Can you work these out from the model? Positions are in its coordinate system, mm. Give positions to 0.01 mm unless a question says otherwise; leave off trailing zeros. Order: outer loops, then holes, each group sorted by start corner. A loop starts at its lowest first (then second) coordinate and runs counter-clockwise, first axis right, second up. Notation, with made-up numbers: M -16.5,40 L 33.5,40 A21 ccw 33.5,75 Z; hole C 59,-30 d7. An arc over 180 degrees is marked long. Write each question's results on one line, items separated by ' | '.
from build123d import *

# Parameters (mm, degrees)
SKETCH1_W           = 34
SKETCH1_H           = 26
BOSS_EXTRUDE1_DEPTH = 1.5
SKETCH2_R           = 1.5
CUT_EXTRUDE1_DEPTH  = 1.5
CHAMFER1_SIZE       = 1


with BuildPart() as part:
    # Sketch1 → Boss-Extrude1 (new body)
    with BuildSketch(Plane(origin=(0, 0, 0), x_dir=(1, 0, 0), z_dir=(0, 1, 0))):
        Rectangle(SKETCH1_W, SKETCH1_H)
    extrude(amount=BOSS_EXTRUDE1_DEPTH)

    # Sketch2 → Cut-Extrude1 (cut)
    with BuildSketch(Plane(origin=(0, 1.5, 0), x_dir=(1, 0, 0), z_dir=(0, 1, 0))):
        with Locations(Location((-14.5, 10.5, 0), (0, 0, 270))):
            Circle(SKETCH2_R)
        with Locations(Location((11.5, 10.5, 0), (0, 0, 270))):
            Circle(SKETCH2_R)
        with Locations(Location((11.5, -10.5, 0), (0, 0, 270))):
            Circle(SKETCH2_R)
        with Locations(Location((-14.5, -10.5, 0), (0, 0, 270))):
            Circle(SKETCH2_R)
    extrude(amount=-CUT_EXTRUDE1_DEPTH, mode=Mode.SUBTRACT)

    # Chamfer1
    chamfer1_edges = [part.edges().sort_by_distance(p)[0] for p in [
        (17, 0.75, 13),
        (-17, 0.75, 13),
        (-17, 0.75, -13),
        (17, 0.75, -13),
    ]]
    chamfer(chamfer1_edges, length=CHAMFER1_SIZE)


solid = part.part
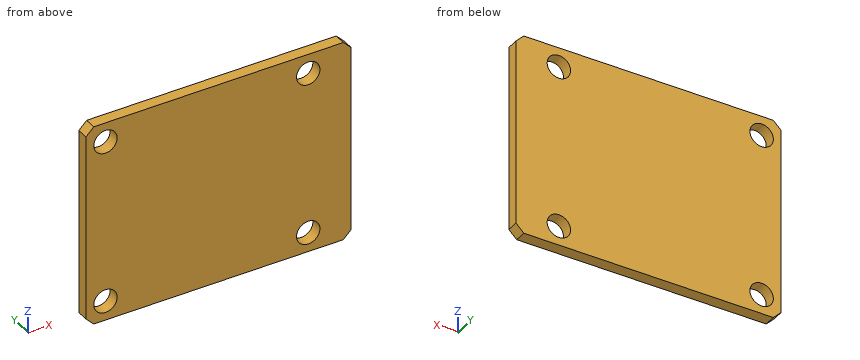
(1) Imagine slicing it at A-A, the plane z = 10.5. Write out the boundary of the cut face in (x, y).
Data:
outline: M -17,0 L -16,0 L -16,1.5 L -17,1.5 Z; M -13,0 L 10,0 L 10,1.5 L -13,1.5 Z; M 13,0 L 17,0 L 17,1.5 L 13,1.5 Z
(2) Imagine slicing it at C-C, the plane x = -14.5. Write out the boundary of the cut face in (y, z).
Data:
outline: M 0,-13 L 1.5,-13 L 1.5,-12 L 0,-12 Z; M 0,-9 L 1.5,-9 L 1.5,9 L 0,9 Z; M 0,12 L 1.5,12 L 1.5,13 L 0,13 Z
(3) I need wall thicknesses on L1, parallel to X at y = 0.85, z = -10.5; L2, parallel to X at y = 1.2, z = 11; L3, parallel to Z at x = -13.5, y = 0.7. Which ranges of each line are inside material? Lowest first, please. Write a range as from..to.
Data:
L1: x = -17..-16, -13..10, 13..17 | L2: x = -17..-15.91, -13.09..10.09, 12.91..17 | L3: z = -13..-11.62, -9.38..9.38, 11.62..13
(4) Imagine slicing it at B-B, the plane y = 0.9. Write out the boundary of the cut face in (x, z), plus the area to 3 significant figures.
Data:
outline: M -17,-12 L -16,-13 L 16,-13 L 17,-12 L 17,12 L 16,13 L -16,13 L -17,12 Z; hole C -14.5,-10.5 d3; hole C -14.5,10.5 d3; hole C 11.5,-10.5 d3; hole C 11.5,10.5 d3 | area: 854 mm2
